Geometry check sheet. Reference: drawing and pictorial views, mm from the part's lowest x, y, z. A direction names the side the tool comes from. Coordinates: 2 decimals unless noted, no trailing zeros. Loops run counter-clockwise (first coordinate to the right, second up) from the corner with the lowest first, then second, coordinate; pieces in that order, holes last. Notation, with made-up numbers: (46, -30) -> (50, -30) arc R30 ccw to (50, -4) -> close; hole circle Ø2 at (-27, 5.25). An arc over 180 degrees is marked (long way). Use CSV: the item, a comma, the result in double quotes.
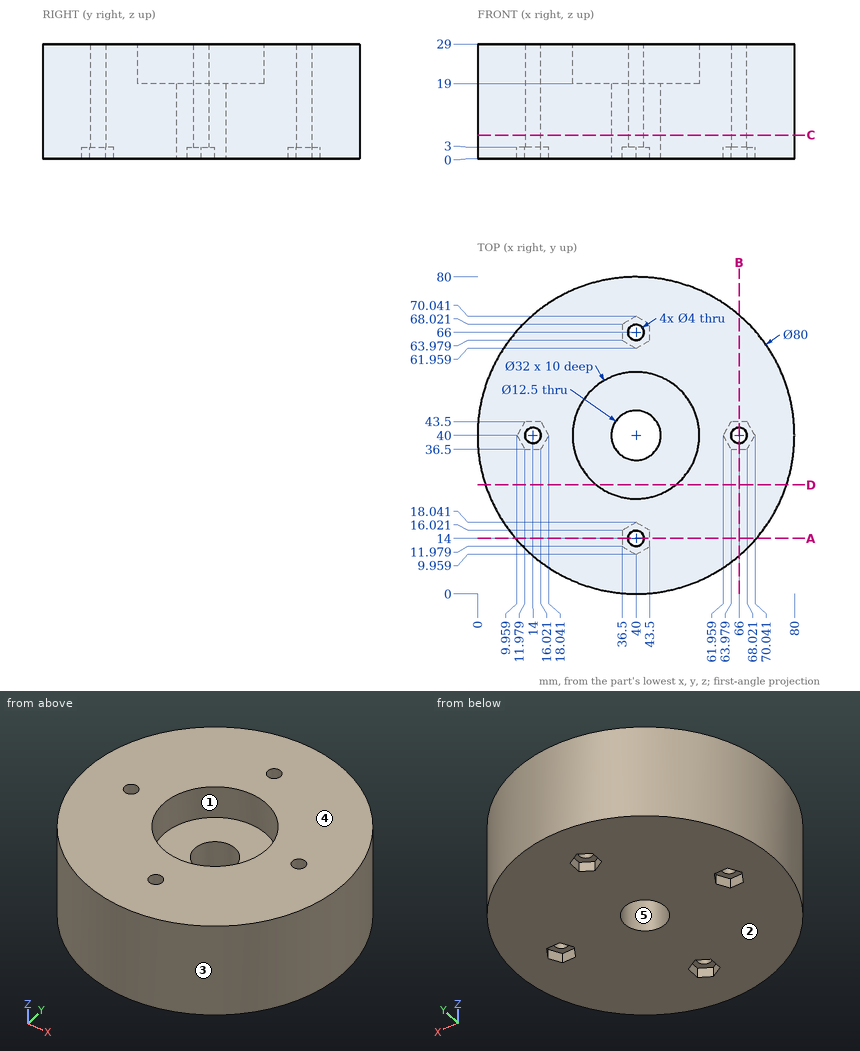
1) Cross-section at C-C on z = 6. Record the boundary of the cut face in (x, y), and give its area (3 significant figures).
Answer below:
outline,"circle Ø80 at (40, 40); hole circle Ø4 at (14, 40); hole circle Ø12.5 at (40, 40); hole circle Ø4 at (40, 14); hole circle Ø4 at (40, 66); hole circle Ø4 at (66, 40)"
area,"4,850 mm²"
2) Access from +Z, -Z, +X, -X, +Y, -Y to the whole of each face (thin tool, end or side, straight path). Record for the marked faces 1 and 2.
Answer below:
face 1,"+Z"
face 2,"-Z, +X, -X, +Y, -Y"
3) Thickness scan on line 1 along Y through (x, z) = (40, 21.75); line 2 along Y through (x, z) = (40, 16.25); line 3 along Y through (x, z) = (66, 9.5) (1 decimal). Record the ranges inside material, lowest first. Write a range as from..to.
Answer below:
line 1,"y = 0..12, 16..24, 56..64, 68..80"
line 2,"y = 0..12, 16..33.75, 46.25..64, 68..80"
line 3,"y = 9.6..38, 42..70.4"
4) Cross-section at D-D on y = 27.5. Record the boundary of the cut face in (x, z).
Answer below:
outline,"(2, 0) -> (78, 0) -> (78, 29) -> (49.99, 29) -> (49.99, 19) -> (30.01, 19) -> (30.01, 29) -> (2, 29) -> close"
5) Draft check along X on the marked faces 3, 4 and 5. Enter one of: released by +X, released by -X, zero draft, split by the parting line, or undercut.
Answer below:
face 3,"split by the parting line"
face 4,"zero draft"
face 5,"undercut"
6) Cross-section at A-A on y = 14. Record the boundary of the cut face in (x, z), and give its area (3 significant figures).
Answer below:
outline,"(9.6, 0) -> (36.5, 0) -> (36.5, 3) -> (38, 3) -> (38, 29) -> (9.6, 29) -> close; (42, 3) -> (43.5, 3) -> (43.5, 0) -> (70.4, 0) -> (70.4, 29) -> (42, 29) -> close"
area,"1,640 mm²"
7) Go/stop test with flat-tipped pins: pin 1 Ø3.5 at (x, y) = (66.5, 39) entering from -Z; pin 2 Ø5 at (x, z) = (50.5, 14) entering from +Y; pin 3 Ø3.5 at (y, z) = (66, 2) entering from -X; pin 4 Ø2.5 at (x, y) = (14, 40) entering from +Z. Record where each tip stops, or that it passes through.
Answer below:
pin 1,"stops at z = 3"
pin 2,"stops at y = 79.19"
pin 3,"stops at x = 8.19"
pin 4,"passes through"
